Geometry: final body of the model. Coordinates: model frame, mm. Give positions to 0.01 mm unless a question says otherwise; leave off trailing zeros. Write each loop counter-clockwise with the first axis right and the second up, starting at its lowest first coordinate (ties: lowest second). Pieces come first, ordered by that corner, then holes. Notation, with made-up numbers: M 84.5,72 L 103.5,72 A15 cw 103.5,99 Z; hole C 4.25,82 d9. An arc over 180 degrees is marked long. One line per question, with ' | ' between items.
from build123d import *

# Parameters (mm, degrees)
SKETCH1_W           = 539.75
SKETCH1_H           = 609.6
BOSS_EXTRUDE1_DEPTH = 25.4
CUT_EXTRUDE1_DEPTH  = 26.4


with BuildPart() as part:
    # Sketch1 → Boss-Extrude1 (new body)
    with BuildSketch(Plane.XY):
        Rectangle(SKETCH1_W, SKETCH1_H)
    extrude(amount=BOSS_EXTRUDE1_DEPTH)

    # Sketch2 → Cut-Extrude1 (cut, through all)
    with BuildSketch(Plane(origin=(0, 0, 0), x_dir=(-1, 0, 0), z_dir=(0, 0, -1))):
        with BuildLine():
            Line((-266.7, -254), (-266.7, 228.6))
            ThreePointArc((-266.7, 228.6), (-251.821024484, 264.521024484), (-215.9, 279.4))
            Line((-215.9, 279.4), (215.9, 279.4))
            ThreePointArc((215.9, 279.4), (251.821024484, 264.521024484), (266.7, 228.6))
            Line((266.7, 228.6), (266.7, -254))
            ThreePointArc((266.7, -254), (251.821024484, -289.921024484), (215.9, -304.8))
            Line((215.9, -304.8), (-215.9, -304.8))
            ThreePointArc((-215.9, -304.8), (-251.821024484, -289.921024484), (-266.7, -254))
        make_face()
    extrude(amount=-CUT_EXTRUDE1_DEPTH, mode=Mode.SUBTRACT)


solid = part.part
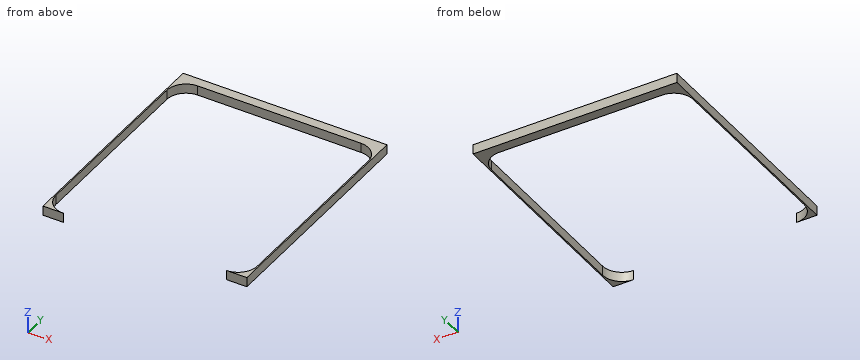
(1) Material intervals for L1, parallel to X at y = 113, z = 21.5 (3 decimals); L2, parallel to Y at x = -15.5, z = 5.5; L3, parallel to X at y = -265.5, z = 5.75 (3 decimals), sorted ascending. Write a range as [from, to].
Working result:
L1: x = [-269.875, -266.7], [266.7, 269.875] | L2: y = [279.4, 304.8] | L3: x = [-269.875, -265.381], [265.381, 269.875]
(2) Cut plane A-A, the plane y = 150.5. Return loops of the section in (x, z) (3 decimals).
Working result:
outline: M -269.875,0 L -266.7,0 L -266.7,25.4 L -269.875,25.4 Z; M 266.7,0 L 269.875,0 L 269.875,25.4 L 266.7,25.4 Z
(3) Cut plane B-B, the plane z = 12. Return loops of the section in (x, y) (3 decimals).
Working result:
outline: M -269.875,-304.8 L -215.9,-304.8 A50.8 cw -266.7,-254 L -266.7,228.6 A50.8 cw -215.9,279.4 L 215.9,279.4 A50.8 cw 266.7,228.6 L 266.7,-254 A50.8 cw 215.9,-304.8 L 269.875,-304.8 L 269.875,304.8 L -269.875,304.8 Z
(4) Cut plane C-C, the plane x = -233. Return loops of the section in (y, z), then the cut area to 3 significant figures.
Working result:
outline: M -304.8,0 L -301.84,0 L -301.84,25.4 L -304.8,25.4 Z; M 276.44,0 L 304.8,0 L 304.8,25.4 L 276.44,25.4 Z | area: 796 mm^2
(5) First-contact query: P1, Ø1.5, axis at x = -144.5, z = 7.5, coming from the -Y side. Flat tip, straight axial feed; report the tip coordinate or a pass-through.
Working result:
P1: stops at y = 279.4
